Geometry check sheet. Reference: the model listing, model coordinates, mm. A direction names the side the tool comes from. Coordinates: 2 decimals unless noted, no trailing zeros. Loops run counter-clockwise (first coordinate to the right, second up) from the corner with the lowest first, then second, coordinate; pieces in that order, holes last. Notation, with made-up numbers: (22.25, 45.25) - (79.25, 45.25) arc R22 cw to (79.25, 60.25) - close; hole circle Ø1 at (-30.5, 80). An arc over 180 degrees is marked (long way). One line per item, written item: value.
from build123d import *

# Parameters (mm, degrees)
F0_W     = 5
F0_H     = 5
F1_DEPTH = 0.1
F2_W     = 40
F2_H     = 40
F3_DEPTH = 1
F4_R     = 0.5
F5_DEPTH = 2


with BuildPart() as f1:
    # F0 (on Top) → F1 (new body)
    with BuildSketch(Plane.XY):
        with Locations((-6, 6)):
            Rectangle(F0_W, F0_H)
        with Locations((6, 6)):
            Rectangle(F0_W, F0_H)
        with Locations((6, -6)):
            Rectangle(F0_W, F0_H)
        with Locations((-6, -6)):
            Rectangle(F0_W, F0_H)
    extrude(amount=-F1_DEPTH)

    # F2 (on Top) → F3 (join)
    with BuildSketch(Plane.XY):
        Rectangle(F2_W, F2_H)
    extrude(amount=F3_DEPTH)

    # F4 (on face) → F5 (join)
    with BuildSketch(Plane(origin=(0, 0, -0.1), x_dir=(1, 0, 0), z_dir=(0, 0, -1))):
        with Locations((-7.090843, 7.180036)):
            Circle(F4_R)
        with Locations((-5.090843, 7.180036)):
            Circle(F4_R)
        with Locations((-7.090843, 4.807855)):
            Circle(F4_R)
        with Locations((-5.090843, 4.807855)):
            Circle(F4_R)
        with Locations((7.090843, 7.180036)):
            Circle(F4_R)
        with Locations((5.090843, 7.180036)):
            Circle(F4_R)
        with Locations((5.090843, 4.807855)):
            Circle(F4_R)
        with Locations((7.090843, 4.807855)):
            Circle(F4_R)
        with Locations((-7.090843, -4.807855)):
            Circle(F4_R)
        with Locations((-5.090843, -7.180036)):
            Circle(F4_R)
        with Locations((-7.090843, -7.180036)):
            Circle(F4_R)
        with Locations((-5.090843, -4.807855)):
            Circle(F4_R)
        with Locations((5.090843, -7.180036)):
            Circle(F4_R)
        with Locations((5.090843, -4.807855)):
            Circle(F4_R)
        with Locations((7.090843, -4.807855)):
            Circle(F4_R)
        with Locations((7.090843, -7.180036)):
            Circle(F4_R)
    extrude(amount=F5_DEPTH)


solid = f1.part
(1) Material ranges on probe 1 along X at (y, z) = (4.5, -0.5); probe 2 along Z at (x, y) = (-6.5, -5); probe 3 along Z at (x, y) = (-13, 4), recorded low to high. Write a range as from..to.
Reply:
probe 1: -7.48..-6.7, -5.48..-4.7, 4.7..5.48, 6.7..7.48
probe 2: -0.1..1
probe 3: 0..1
(2) Cross-section at C-C on y = -10. Record the cut outline in (x, z), and give its area (3 significant figures).
Reply:
outline: (-20, 0) - (20, 0) - (20, 1) - (-20, 1) - close
area: 40.0 mm2
(3) Cross-section at B-B on x = 4. Record the cut outline in (y, z), and give its area (3 significant figures).
Reply:
outline: (-20, 0) - (-8.5, 0) - (-8.5, -0.1) - (-3.5, -0.1) - (-3.5, 0) - (3.5, 0) - (3.5, -0.1) - (8.5, -0.1) - (8.5, 0) - (20, 0) - (20, 1) - (-20, 1) - close
area: 41.0 mm2
(4) Access from +Z, -Z, +X, -X, +Y, -Y to the whole of each face (thin tool, end or side, straight path). Record for faces 1 (the face through (-7, -7, -2.1)), 2 (the face through (5.553, 7.372, -1.086)).
Reply:
face 1: -Z, +X, -X, +Y, -Y
face 2: -Z
(5) Release check for a two-part mould opening along X. For faces 3 (the face through (20, -0.3, 0.5)), 4 (the face through (5, -7, -2.1)), 5 (the face through (6, -6, -0.1)) record: pulls with the +X half, pulls with the -X half, needs draft (parallel to the pull), parting line crosses it, or undercut.
Reply:
face 3: pulls with the +X half
face 4: needs draft
face 5: undercut
(6) Go/stop test with a flat-tipped pin: pin 1 Ø4 at (x, y) = (12, -7.5) entering from -Z. Record where the tip stops, or that it passes through.
Reply:
pin 1: z = 0
(7) Cross-section at A-A on z = -1.35. State how many separate pieces and enclosed holes the cut face has, and give its area (3 significant figures).
Reply:
separate pieces: 16
enclosed holes: 0
area: 12.6 mm2
